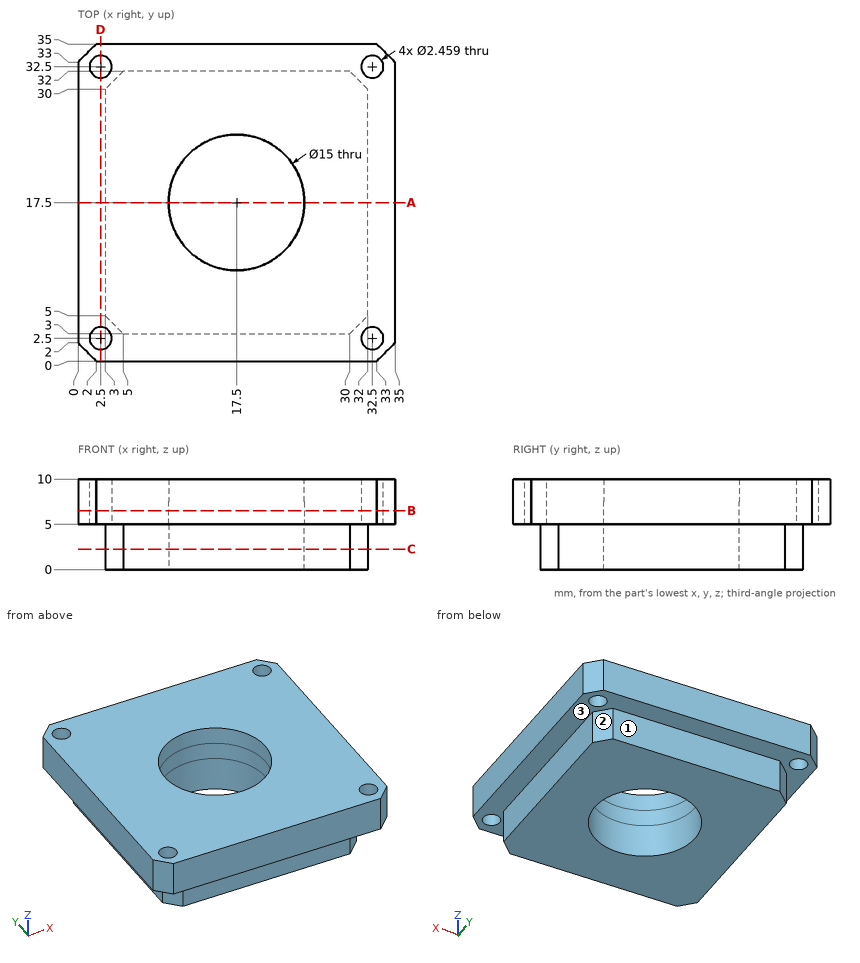
For this review, use the dimensioned drawing (mm, ordinates from the lowest corner) and the shaded views. A direction names the side the tool comes from. Coordinates: 2 decimals unless noted, no trailing zeros. Write each loop counter-clockwise with the first axis right and the second up, starting at its lowest first coordinate (ties: lowest second). Pieces come first, ordered by that corner, then holes. Notation, with made-up numbers: (0.5, 62.5) - (51.5, 62.5) arc R10 ccw to (51.5, 75.5) - close; hole circle Ø4 at (77.5, -38). An arc over 180 degrees is marked (long way). Answer in a Markdown table with one row per item. Add a question column.
Q1. Consider section C-C on z = 2.25. Give the boundary of the cut face in (x, y), then the cut area to 3 significant figures.
Q2. Clearance check with flat-ended pins moving along their axes: pin 1 (1.5 mm diameter, centred on y = 12, z = 1.5, fed in from -X); pin 2 (1.5 mm diameter, centred on x = 19, z = 2, fed in from +Y); pin 3 (3 mm diameter, centred on x = 2.5, y = 32.5, fed in from -Z). State where each tip first meets the part, or that it passes through.
Q3. Consider section B-B on z = 6.5. Give the boundary of the cut face in (x, y), then the cut area to 3 significant figures.
Q4. To check wall thickness, follow line 1 along Y through (x, z) = (32.5, 6.55); line 2 along Y through (x, z) = (17.5, 9.1). State the ranges of each line that lie inside material, in increasing order. Write a range as from..to.
Q5. For the marked faces 1, 2 and 3, list the 3-axis set-ups (+Z, -Z, +X, -X, +Y, -Y) from which the entire face can be reached by the end or side of a thin tool; tool diameter is ignored.
Q6. Consider section A-A on y = 17.5. Give the boundary of the cut face in (x, z), then the cut area to 3 significant figures.
Q7. Consider section D-D on x = 2.5. Give the boundary of the cut face in (y, z).
Answers below:
| question | item | result |
|---|---|---|
| 1 | outline | (3, 5) - (5, 3) - (30, 3) - (32, 5) - (32, 30) - (30, 32) - (5, 32) - (3, 30) - close; hole circle Ø15 at (17.5, 17.5) |
| 1 | area | 656 mm² |
| 2 | pin 1 | x = 3 |
| 2 | pin 2 | y = 32 |
| 2 | pin 3 | z = 5 |
| 3 | outline | (0, 2) - (2, 0) - (33, 0) - (35, 2) - (35, 33) - (33, 35) - (2, 35) - (0, 33) - close; hole circle Ø2.46 at (2.5, 2.5); hole circle Ø2.46 at (2.5, 32.5); hole circle Ø15 at (17.5, 17.5); hole circle Ø2.46 at (32.5, 2.5); hole circle Ø2.46 at (32.5, 32.5) |
| 3 | area | 1,020 mm² |
| 4 | line 1 | 0..1.27, 3.73..31.27, 33.73..35 |
| 4 | line 2 | 0..10, 25..35 |
| 5 | face 1 | -Z, +X, -X, +Y |
| 5 | face 2 | -Z, +X, +Y |
| 5 | face 3 | -Z |
| 6 | outline | (0, 5) - (3, 5) - (3, 0) - (10, 0) - (10, 10) - (0, 10) - close; (25, 0) - (32, 0) - (32, 5) - (35, 5) - (35, 10) - (25, 10) - close |
| 6 | area | 170 mm² |
| 7 | outline | (0, 5) - (1.27, 5) - (1.27, 10) - (0, 10) - close; (3.73, 5) - (31.27, 5) - (31.27, 10) - (3.73, 10) - close; (33.73, 5) - (35, 5) - (35, 10) - (33.73, 10) - close |
